Can you work these out from the drawing? Everything is in mm from the part's minimum corner. Give positions to 0.01 mm unless a question says otherwise; leave off trailing zeros. Order: outer loops, then holes, each group sorted by start corner. A loop starts at its lowest first (then second) coordinate and runs counter-clockwise, first axis right, second up. Notation, with made-up numbers: M -27,47 L 30,47 A21 cw 30,64 Z; hole C 11,86.5 d7. An arc over 180 degrees is marked long. Answer as a JSON object with one key per item and string values.
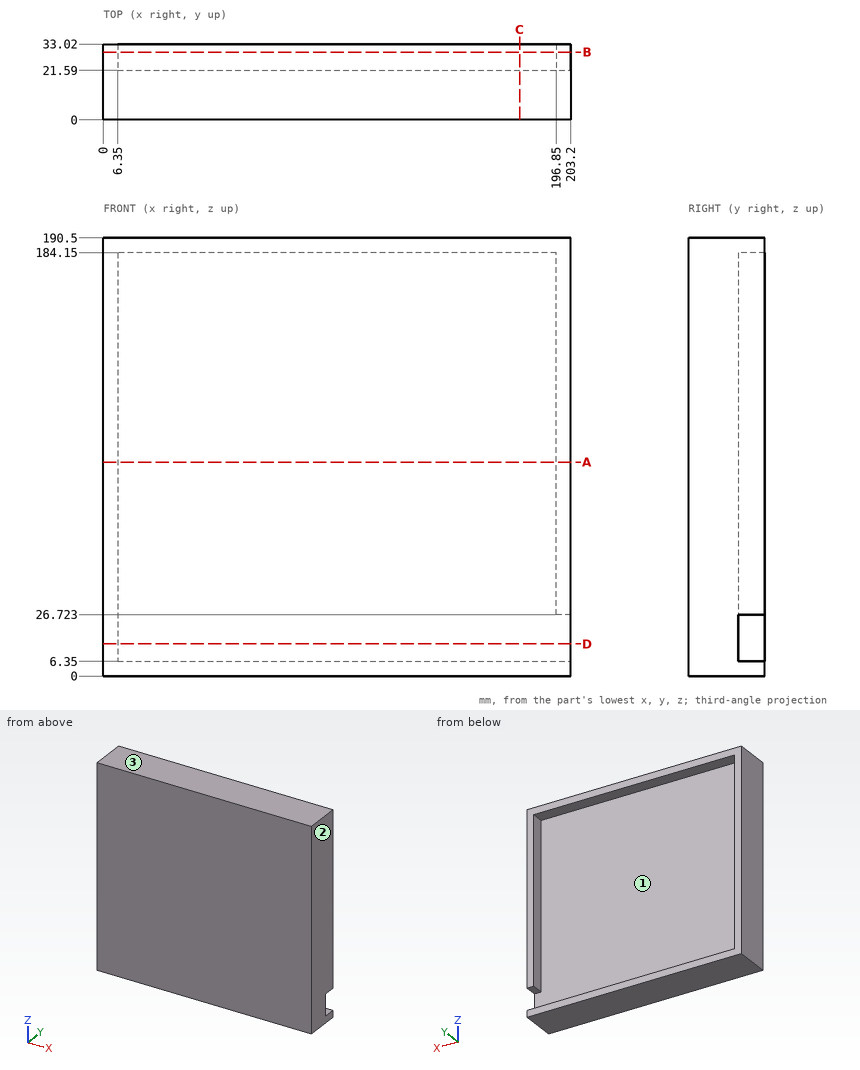
1) I want a section at C-C on x = 181. Write out the boundary of the cut face in (y, z), and give its area (3 significant figures).
Results found:
{"outline": "M 0,0 L 33.02,0 L 33.02,6.35 L 21.59,6.35 L 21.59,184.15 L 33.02,184.15 L 33.02,190.5 L 0,190.5 Z", "area": "4,260 mm²"}
2) I'm going to push a flat-ended pin straight in: pin 1 Ø4 at (x, z) = (133, 48.5) entering from +Y. Where does the tip first touch, or does it pass through?
Results found:
{"pin 1": "stops at y = 21.59"}
3) I want a section at B-B on y = 29.5. Write out the boundary of the cut face in (x, z).
Results found:
{"outline": "M 0,0 L 203.2,0 L 203.2,6.35 L 6.35,6.35 L 6.35,184.15 L 196.85,184.15 L 196.85,26.72 L 203.2,26.72 L 203.2,190.5 L 0,190.5 Z"}
4) I want a section at D-D on z = 14. Write out the boundary of the cut face in (x, y).
Results found:
{"outline": "M 0,0 L 203.2,0 L 203.2,21.59 L 6.35,21.59 L 6.35,33.02 L 0,33.02 Z"}
5) Thinking about a two-plate mould opening in Z: for the marked faces 1, 2 and 3, which applies, pulls with the +Z half, pulls with the -Z half, needs draft (parallel to the pull), parting line crosses it, or undercut?
Results found:
{"face 1": "undercut", "face 2": "needs draft", "face 3": "pulls with the +Z half"}
6) I need wall thicknesses on L1, parallel to X at y = 22, z = 48; L2, parallel to Z at x = 96.5, y = 31.5; L3, parallel to Y at x = 134, z = 176. Which ranges of each line are inside material? Lowest first, please.
Results found:
{"L1": "x = 0 to 6.35, 196.85 to 203.2", "L2": "z = 0 to 6.35, 184.15 to 190.5", "L3": "y = 0 to 21.59"}
7) I want a section at A-A on z = 93. Write out the boundary of the cut face in (x, y).
Results found:
{"outline": "M 0,0 L 203.2,0 L 203.2,33.02 L 196.85,33.02 L 196.85,21.59 L 6.35,21.59 L 6.35,33.02 L 0,33.02 Z"}
